Model file for the job. Use its own axes, mm. A direction names the side the tool comes from. Give positions to 0.01 mm unless a question says otherwise; leave off trailing zeros. Write each loop counter-clockwise with the first axis right and the second up, starting at its lowest first coordinate (ties: lowest second). Pieces come first, ordered by that corner, then holes.
```python
from build123d import *

# Parameters (mm, degrees)
ESQUISSE2_R             = 2
ENL_V_MAT_EXTRU_1_DEPTH = 10


with BuildPart() as part:
    # Esquisse1 → Révolution1 (revolve)
    with BuildSketch(Plane.XY):
        Polygon((0, 0), (0, 9), (0.5, 9), (1, 8), (3, 8), (3.5, 9), (4, 9), (7, 9), (7, 0), (4, 0), align=None)
    revolve(axis=Axis((4, 0, 0), (-1, 0, 0)))

    # Esquisse2 → Enlèv. mat.-Extru.1 (cut)
    with BuildSketch(Plane.ZY):
        with Locations(Location((0, 5.95, 0), (0, 0, 270))):
            Circle(ESQUISSE2_R)
        with Locations(Location((5.95, 0, 0), (0, 0, 270))):
            Circle(ESQUISSE2_R)
        with Locations(Location((0, -5.95, 0), (0, 0, 270))):
            Circle(ESQUISSE2_R)
        with Locations(Location((-5.95, 0, 0), (0, 0, 270))):
            Circle(ESQUISSE2_R)
    extrude(amount=-ENL_V_MAT_EXTRU_1_DEPTH, mode=Mode.SUBTRACT)


solid = part.part
```
1. Slice it at B-B, the plane x = 3.25. Write the cut outline in (y, z).
Calculated:
outline: circle Ø17 at (0, 0); hole circle Ø4 at (-5.95, 0); hole circle Ø4 at (0, -5.95); hole circle Ø4 at (0, 5.95); hole circle Ø4 at (5.95, 0)
2. Slice it at A-A, the plane x = 1.75. Write the cut outline in (y, z).
Calculated:
outline: circle Ø16 at (0, 0); hole circle Ø4 at (-5.95, 0); hole circle Ø4 at (0, -5.95); hole circle Ø4 at (0, 5.95); hole circle Ø4 at (5.95, 0)
3. Slice it at C-C, the plane z = -1.5. State how many separate pieces and enclosed holes the cut face has, and give its area (3 significant figures).
Calculated:
separate pieces: 3
enclosed holes: 0
area: 82.1 mm2
4. Which spindle directions (+Z, -Z, +X, -X, +Y, -Y) get a long thin tool onto all of the face, cutting with end or side? Do faces 1 (the cylindrical face through (2.01, -1.73, 7.81)), 2 (the cylindrical face through (3.451, -7.797, -0.766)). Say none if no direction does.
Calculated:
face 1: none
face 2: +X, -X
5. Probe probe 1 along Z at (x, y) = (4.5, 0); probe 2 along Y at (x, z) = (4.5, -1); probe 3 along Y at (x, z) = (6, -5). List the from-to ranges inside material, lowest first.
Calculated:
probe 1: z = -9 to -7.95, -3.95 to 3.95, 7.95 to 9
probe 2: y = -8.94 to -7.68, -4.22 to 4.22, 7.68 to 8.94
probe 3: y = -7.48 to -1.76, 1.76 to 7.48
6. Pull direction Y, two halves, no side cores. Call faces 3 (the cylindrical face through (0.254, -1.172, -8.923)), 4 (the cylindrical face through (3, 6, -2)), 5 (the flat face through (7, 0, 0)): +Y half, -Y half, draft (parallel to the pull), parting line (faces both ways), or undercut.
Calculated:
face 3: parting line
face 4: undercut
face 5: draft
7. Pin check, flat tips, straight feed: P1, Ø4, axis at x = 5.5, y = 2.5, coming from the +Z side; P2, Ø1.5, axis at x = 2, y = -7, coming from the +Z side. Stop position of each tip, or through.
Calculated:
P1: stops at z = 8.99
P2: stops at z = 4.99
